Source: three-view drawing plus pictorial views. Frame: mm from the lowest corner of the part. A direction names the side the tool comes from. Give positions to 0.01 mm unless a question says otherwise; leave off trailing zeros. Order: outer loops, then holes, each group sorted by start corner. A loop starts at its lowest first (then second) coordinate and runs counter-clockwise, first axis right, second up.
1) Material intervals for line 1 (Y direction, x = 12.55, z = 7); line 2 (Y direction, x = 13.2, z = 7); line 3 (Z direction, x = 10, y = 4.25), sorted ascending.
2) Draft query along Y for the marked faces 3, 4 and 5. Return one class per face: released by +Y, released by -Y, zero draft, split by the parting line, or undercut.
3) Access query for the marked faces 1 and 2. Directions: +Z, -Z, +X, -X, +Y, -Y. A direction counts if a zero-diameter tool reaches every point of the face in a straight line with its end or side. Return the directions, or none.
4) Section A-A, the plane z = 37. Return loops of the section in (x, y).
5) Section D-D, the plane y = 3. Return loops of the section in (x, z).
6) Section C-C, the plane y = 18. Return loops of the section in (x, z), plus the area to 3 significant figures.
7) Section B-B, the plane y = 10. Return loops of the section in (x, z).
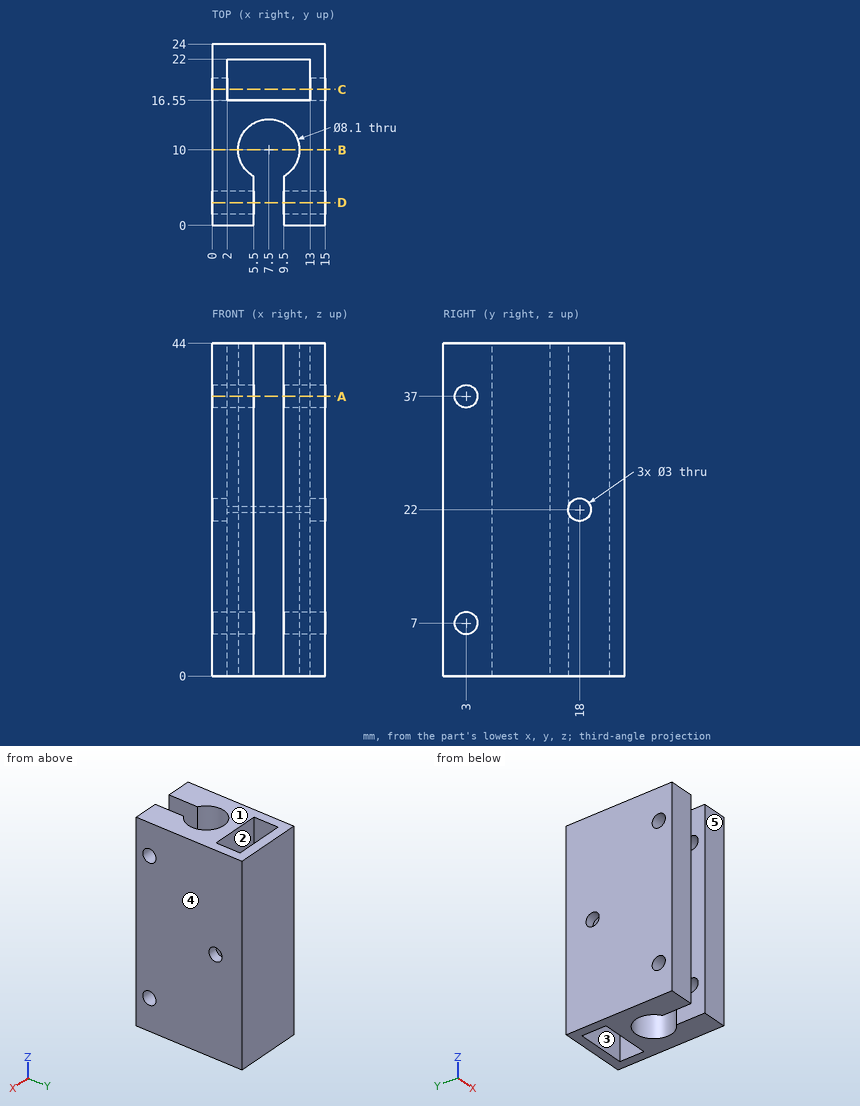
From the geometry:
1. line 1: y = 0 to 1.5, 4.5 to 16.55, 22 to 24
1. line 2: y = 0 to 1.5, 4.5 to 24
1. line 3: z = 0 to 6.17, 7.83 to 36.17, 37.83 to 44
2. face 3: undercut
2. face 4: zero draft
2. face 5: released by -Y
3. face 1: +Z, +X, -X, +Y, -Y
3. face 2: +Z, -Z
4. outline: (0, 0) - (5.5, 0) - (5.5, 1.5) - (0, 1.5) - close; (0, 4.5) - (5.5, 4.5) - (5.5, 6.48) arc R4.05 cw (long way) to (9.5, 6.48) - (9.5, 4.5) - (15, 4.5) - (15, 24) - (0, 24) - close; (9.5, 0) - (15, 0) - (15, 1.5) - (9.5, 1.5) - close; hole (2, 16.55) - (13, 16.55) - (13, 22) - (2, 22) - close
5. outline: (0, 0) - (5.5, 0) - (5.5, 5.5) - (0, 5.5) - close; (0, 8.5) - (5.5, 8.5) - (5.5, 35.5) - (0, 35.5) - close; (0, 38.5) - (5.5, 38.5) - (5.5, 44) - (0, 44) - close; (9.5, 0) - (15, 0) - (15, 5.5) - (9.5, 5.5) - close; (9.5, 8.5) - (15, 8.5) - (15, 35.5) - (9.5, 35.5) - close; (9.5, 38.5) - (15, 38.5) - (15, 44) - (9.5, 44) - close
6. outline: (0, 0) - (2, 0) - (2, 20.5) - (0, 20.5) - close; (0, 23.5) - (2, 23.5) - (2, 44) - (0, 44) - close; (13, 0) - (15, 0) - (15, 20.5) - (13, 20.5) - close; (13, 23.5) - (15, 23.5) - (15, 44) - (13, 44) - close
6. area: 164 mm2
7. outline: (0, 0) - (3.45, 0) - (3.45, 44) - (0, 44) - close; (11.55, 0) - (15, 0) - (15, 44) - (11.55, 44) - close
